from build123d import *

# Parameters (mm, degrees)
CUT_EXTRUDE2_START  = -7
SKETCH4_R           = 5
SKETCH4_R_2         = 3.9
CUT_EXTRUDE2_DEPTH  = 7
SKETCH3_R           = 5
SKETCH3_R_2         = 3.9
CUT_EXTRUDE4_DEPTH  = 12
SKETCH7_R           = 6.25
BOSS_EXTRUDE1_DEPTH = 5
BOSS_EXTRUDE2_DEPTH = 5
CIRPATTERN1_COUNT   = 12


with BuildPart() as part:
    # Sketch2 → Revolve1 (revolve)
    with BuildSketch(Plane(origin=(0, 0, 0), x_dir=(1, 0, 0), z_dir=(0, 1, 0))):
        Polygon((40, -5), (-40, -5), (-40, 0), (-30.049059985, 0), (-24.904700538, 0), (-23.75, -2), (-21.25, -2), (-20.095299462, 0), (-9.904700538, 0), (-8.75, -2), (-6.25, -2), (-5.095299462, 0), (5.095299462, 0), (6.25, -2), (8.75, -2), (9.904700538, 0), (20.095299462, 0), (21.25, -2), (23.75, -2), (24.904700538, 0), (30.049059985, 0), (40, 0), align=None)
    revolve(axis=Axis((40, 0, 5), (-1, 0, 0)))

    # Sketch4 → Cut-Extrude2 (cut)
    with BuildSketch(Plane.ZY.offset(40).offset(CUT_EXTRUDE2_START)):
        with Locations(Location((5, 0, 0), (0, 0, 180))):
            Circle(SKETCH4_R)
        with Locations((5, 0)):
            Circle(SKETCH4_R_2, mode=Mode.SUBTRACT)
    extrude(amount=CUT_EXTRUDE2_DEPTH, mode=Mode.SUBTRACT)

    # Sketch3 → Cut-Extrude4 (cut)
    with BuildSketch(Plane(origin=(40, 0, 0), x_dir=(0, 0, -1), z_dir=(1, 0, 0))):
        with Locations((-5, 0)):
            Circle(SKETCH3_R)
        with Locations(Location((-5, 0, 0), (0, 0, 180))):
            Circle(SKETCH3_R_2, mode=Mode.SUBTRACT)
    extrude(amount=-CUT_EXTRUDE4_DEPTH, mode=Mode.SUBTRACT)

    # Sketch7 → Boss-Extrude1 (add)
    with BuildSketch(Plane(origin=(40, 0, 0), x_dir=(0, 0, -1), z_dir=(1, 0, 0))):
        with Locations((-5, 0)):
            Circle(SKETCH7_R)
    extrude(amount=-BOSS_EXTRUDE1_DEPTH)

    # Sketch6 → Boss-Extrude2 (add)
    with BuildSketch(Plane(origin=(40, 0, 0), x_dir=(0, 0, -1), z_dir=(1, 0, 0))):
        Polygon((-5.8, 7.9), (-4.2, 7.9), (-3.7, 5.7), (-6.3, 5.7), align=None)
    boss_extrude2 = extrude(amount=-BOSS_EXTRUDE2_DEPTH)

    # CirPattern1: Boss-Extrude2 ×12 about axis
    cirpattern1_axis = Axis((0, 0, 5), (1, 0, 0))
    for i in range(1, CIRPATTERN1_COUNT):
        add(boss_extrude2.rotate(cirpattern1_axis, i * 360 / CIRPATTERN1_COUNT))


solid = part.part
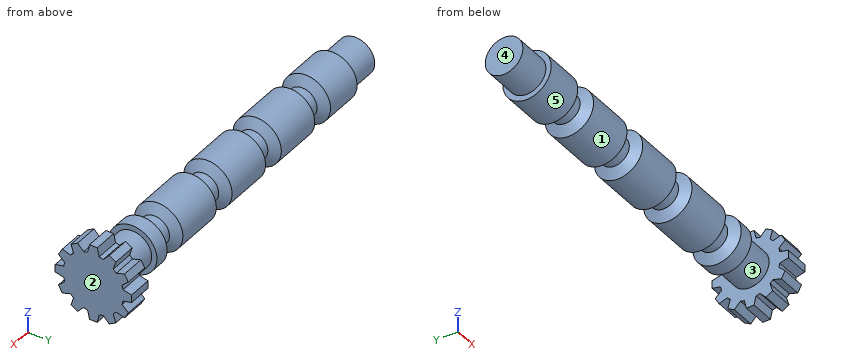
Check sheet for the modelled part. Datum: model origin and axes. Units: mm. Face numbers are marked on the shaded views. A direction names the side the tool comes from. Coordinates: 2 decimals unless noted, no trailing zeros. Write each loop counter-clockwise with the first axis right and the second up, starting at its lowest first coordinate (ties: lowest second). Pieces come first, ordered by that corner, then holes.
Item 1: Mould release check, pull along X, two halves, no side actions. Record for the marked faces 1, 2 and 3: released by +X, released by -X, zero draft, split by the parting line, or undercut.
Numbers:
face 1: zero draft
face 2: released by +X
face 3: undercut
Item 2: Depth check by flat-ended pin: pin 1 Ø6 at (x, z) = (-2.5, 4.5) entering from -Y; pin 2 Ø5 at (x, z) = (-4, 8.5) entering from +Y; pin 3 Ø8 at (x, z) = (-32, 7) entering from +Y. Enter the tip coordinate at first touch or a pass-through.
Numbers:
pin 1: stops at y = -5
pin 2: stops at y = 4.9
pin 3: stops at y = 5
Item 3: Scan lines: probe 1 along X at (y, z) = (3.5, 6.5); probe 2 along X at (y, z) = (-3.5, 3); probe 3 along X at (y, z) = (-2.5, 1.25). Record each from-to range of solid material in increasing order.
Numbers:
probe 1: x = -40 to -24.22, -20.78 to -9.22, -5.78 to 5.78, 9.22 to 20.78, 24.22 to 40
probe 2: x = -33 to -24.35, -20.65 to -9.35, -5.65 to 5.65, 9.35 to 20.65, 24.35 to 28, 35 to 40
probe 3: x = -33 to -24.62, -20.38 to -9.62, -5.38 to 5.38, 9.62 to 20.38, 24.62 to 28, 35 to 40
Item 4: Cross-section at B-B on x = -11. Record the boundary of the cut face in (y, z).
Numbers:
outline: circle Ø10 at (0, 5)
Item 5: Cross-section at A-A on x = 22. Record the boundary of the cut face in (y, z), then the cut area to 3 significant figures.
Numbers:
outline: circle Ø6 at (0, 5)
area: 28.3 mm2
Item 6: Access from +Z, -Z, +X, -X, +Y, -Y to the whole of each face (thin tool, end or side, straight path). Record for the marked faces 4 and 5.
Numbers:
face 4: +Z, -Z, -X, +Y, -Y
face 5: -X
